```python
from build123d import *

# Parameters (mm, degrees)
SKETCH2_W               = 37
SKETCH2_H               = 37
BOSS_EXTRUDE1_DEPTH     = 1220
SKETCH3_W               = 20
SKETCH3_H               = 10
CUT_EXTRUDE1_DEPTH      = 50
SKETCH4_W               = 80
SKETCH4_H               = 2
SKETCH4_W_2             = 2
SKETCH4_H_2             = 6
CUT_EXTRUDE2_DEPTH      = 20
SKETCH5_R               = 10
CUT_EXTRUDE3_DEPTH      = 1222.310771262
CUT_EXTRUDE3_DEPTH_BACK = 1222.310771262
SKETCH6_R               = 3
CUT_EXTRUDE4_DEPTH      = 1222.310771262
SKETCH7_R               = 3
CUT_EXTRUDE5_DEPTH      = 1222.310771262


with BuildPart() as part:
    # Sketch2 → Boss-Extrude1 (new body)
    with BuildSketch(Plane(origin=(0, 0, 0), x_dir=(0, 0, -1), z_dir=(1, 0, 0))):
        with BuildLine():
            Line((0.5, 0), (39.5, 0))
            ThreePointArc((39.5, 0), (39.853553391, 0.146446609), (40, 0.5))
            Line((40, 0.5), (40, 39.5))
            ThreePointArc((40, 39.5), (39.853553391, 39.853553391), (39.5, 40))
            Line((39.5, 40), (0.5, 40))
            ThreePointArc((0.5, 40), (0.146446609, 39.853553391), (0, 39.5))
            Line((0, 39.5), (0, 0.5))
            ThreePointArc((0, 0.5), (0.146446609, 0.146446609), (0.5, 0))
        make_face()
        with Locations((20, 20)):
            Rectangle(SKETCH2_W, SKETCH2_H, mode=Mode.SUBTRACT)
    extrude(amount=BOSS_EXTRUDE1_DEPTH)

    # Sketch3 → Cut-Extrude1 (cut)
    with BuildSketch(Plane(origin=(0, 0, -40), x_dir=(-1, 0, 0), z_dir=(0, 0, -1))):
        with Locations((-1210, 35)):
            Rectangle(SKETCH3_W, SKETCH3_H)
        with Locations((-1210, 5)):
            Rectangle(SKETCH3_W, SKETCH3_H)
        with Locations((-10, 5)):
            Rectangle(SKETCH3_W, SKETCH3_H)
        with Locations((-10, 35)):
            Rectangle(SKETCH3_W, SKETCH3_H)
    extrude(amount=-CUT_EXTRUDE1_DEPTH, mode=Mode.SUBTRACT)

    # Sketch4 → Cut-Extrude2 (cut)
    with BuildSketch(Plane(origin=(0, 0, -40), x_dir=(-1, 0, 0), z_dir=(0, 0, -1))):
        with Locations((-80, 13)):
            Rectangle(SKETCH4_W, SKETCH4_H)
        with Locations((-134, 9)):
            Rectangle(SKETCH4_W_2, SKETCH4_H_2)
        with Locations((-1086, 9)):
            Rectangle(SKETCH4_W_2, SKETCH4_H_2)
        with Locations((-1140, 13)):
            Rectangle(SKETCH4_W, SKETCH4_H)
    extrude(amount=-CUT_EXTRUDE2_DEPTH, mode=Mode.SUBTRACT)

    # Sketch5 → Cut-Extrude3 (cut, two sides)
    with BuildSketch(Plane(origin=(0, 0, -40), x_dir=(-1, 0, 0), z_dir=(0, 0, -1))) as cut_extrude3_sk:
        with Locations(Location((-1020, 20, 0), (0, 0, 180))):
            Circle(SKETCH5_R)
        with Locations(Location((-610, 20, 0), (0, 0, 180))):
            Circle(SKETCH5_R)
        with Locations(Location((-200, 20, 0), (0, 0, 180))):
            Circle(SKETCH5_R)
    extrude(amount=CUT_EXTRUDE3_DEPTH, mode=Mode.SUBTRACT)
    extrude(cut_extrude3_sk.sketch, amount=-CUT_EXTRUDE3_DEPTH_BACK, mode=Mode.SUBTRACT)

    # Sketch6 → Cut-Extrude4 (cut, through all)
    with BuildSketch(Plane.XZ):
        with Locations(Location((1160, -12, 0), (0, 0, 270))):
            Circle(SKETCH6_R)
        with Locations(Location((820, -12, 0), (0, 0, 270))):
            Circle(SKETCH6_R)
        with Locations(Location((400, -12, 0), (0, 0, 270))):
            Circle(SKETCH6_R)
        with Locations(Location((60, -12, 0), (0, 0, 270))):
            Circle(SKETCH6_R)
    extrude(amount=-CUT_EXTRUDE4_DEPTH, mode=Mode.SUBTRACT)

    # Sketch7 → Cut-Extrude5 (cut, through all)
    with BuildSketch(Plane.XZ):
        with Locations(Location((1045, -30.25, 0), (0, 0, 270))):
            Circle(SKETCH7_R)
        with Locations(Location((865, -30.25, 0), (0, 0, 270))):
            Circle(SKETCH7_R)
        with Locations(Location((685, -30.25, 0), (0, 0, 270))):
            Circle(SKETCH7_R)
        with Locations(Location((535, -30.25, 0), (0, 0, 270))):
            Circle(SKETCH7_R)
        with Locations(Location((355, -30.25, 0), (0, 0, 270))):
            Circle(SKETCH7_R)
        with Locations(Location((175, -30.25, 0), (0, 0, 270))):
            Circle(SKETCH7_R)
    extrude(amount=-CUT_EXTRUDE5_DEPTH, mode=Mode.SUBTRACT)


solid = part.part
```
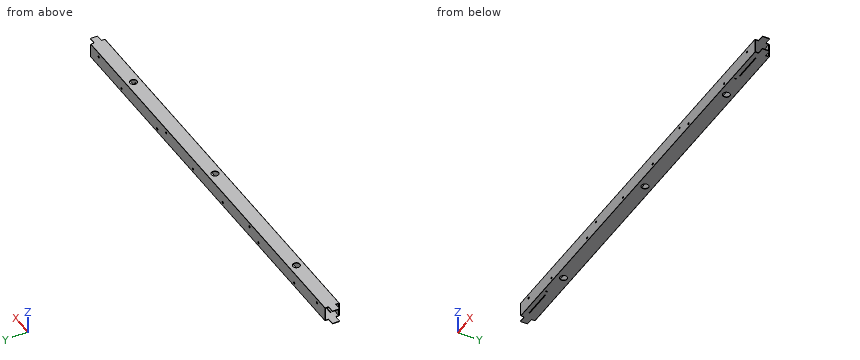
Model file for the job. Use its own axes, mm. Round coordinates to 2 decimals unless told otherwise and drop trailing zeros. Write each loop counter-clockwise with the first axis right and the second up, starting at its lowest first coordinate (ties: lowest second). Pieces come first, ordered by that corner, then holes. Notation, with made-up numbers: (47.25, 81) - (52.25, 81) arc R31 cw to (52.25, 112) - close; hole circle Ø3 at (-35, -36.5). An arc over 180 degrees is marked (long way). Use CSV: the item, a comma, the result in double quotes. Start each with the question number.
Item 1: Band-saw the part on A-A (x = 1062.5). Write the cut outline in (y, z), and give its area (3 significant figures).
Item 2: Band-saw the part on C-C (x = 200). Write the cut outline in (y, z), and give its area (3 significant figures).
Item 3: Pin check, flat tips, straight feed: P1, Ø8, axis at y = 3, z = -22, coming from the -X side; P2, Ø1.2, axis at x = 1210, z = -0.5, coming from the -Y side; P3, Ø11, axis at y = 4, z = -11.5, coming from the +X side. Stop position of each tip, or through.
Item 4: Drill centre lines: L1, parallel to X at y = 39.45, z = -12; L2, parallel to Z at x = 175, y = 39; L3, parallel to Y at x = 1020, z = -0.9. Where is each one in solid material? Low to high. Write a range as [from, to].
Item 5: Band-saw the part on B-B (y = 20). State how many separate pieces and enclosed holes the cut face has, and give its area (3 significant figures).
Checked values:
1,outline,"(0, -39.5) arc R0.5 ccw to (0.5, -40) - (39.5, -40) arc R0.5 ccw to (40, -39.5) - (40, -0.5) arc R0.5 ccw to (39.5, 0) - (0.5, 0) arc R0.5 ccw to (0, -0.5) - close; hole (1.5, -38.5) - (38.5, -38.5) - (38.5, -1.5) - (1.5, -1.5) - close"
1,area,"231 mm²"
2,outline,"(0, -39.5) arc R0.5 ccw to (0.5, -40) - (10, -40) - (10, -38.5) - (1.5, -38.5) - (1.5, -1.5) - (10, -1.5) - (10, 0) - (0.5, 0) arc R0.5 ccw to (0, -0.5) - close; (30, -40) - (39.5, -40) arc R0.5 ccw to (40, -39.5) - (40, -0.5) arc R0.5 ccw to (39.5, 0) - (30, 0) - (30, -1.5) - (38.5, -1.5) - (38.5, -38.5) - (30, -38.5) - close"
2,area,"171 mm²"
3,P1,"stops at x = 20"
3,P2,"stops at y = 10"
3,P3,"stops at x = 1200"
4,L1,"x = [20, 57], [63, 397], [403, 817], [823, 1157], [1163, 1200]"
4,L2,"z = [-40, -33.25], [-27.25, 0]"
4,L3,"y = [0, 10], [30, 40]"
5,separate pieces,"8"
5,enclosed holes,"0"
5,area,"3,480 mm²"
